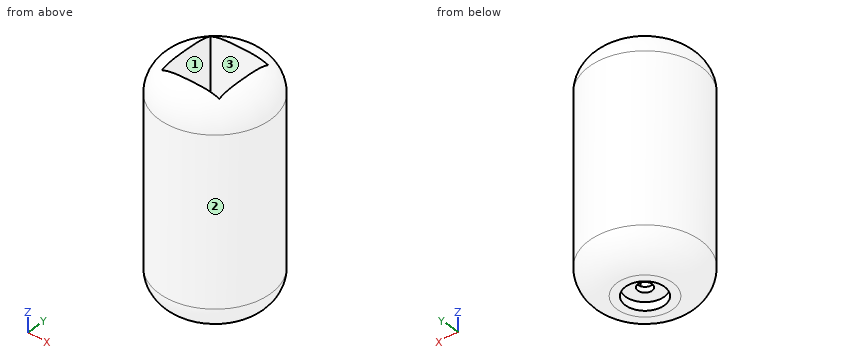
```python
from build123d import *

# Parameters (mm, degrees)
SKETCH4_R               = 20
BODY_DEPTH              = 80
CUT_EXTRUDE1_DEPTH      = 50
CUT_EXTRUDE1_DEPTH_BACK = 50
SKETCH16_W              = 21
SKETCH16_H              = 21
SKETCH17_R              = 2.55
CUT_EXTRUDE2_DEPTH      = 55
SKETCH18_R              = 7
CUT_EXTRUDE3_DEPTH      = 3
FILLET1_R               = 10


with BuildPart() as part:
    # Sketch4 → Body (new body)
    with BuildSketch(Plane.XY.offset(25)):
        Circle(SKETCH4_R)
    extrude(amount=-BODY_DEPTH)

    # Sketch16 → Cut-Extrude1 (cut, two sides: drawn at the far end of the back side and taken through both)
    with BuildSketch(Plane.XY.offset(-CUT_EXTRUDE1_DEPTH_BACK)):
        Rectangle(SKETCH16_W, SKETCH16_H)
    extrude(amount=CUT_EXTRUDE1_DEPTH + CUT_EXTRUDE1_DEPTH_BACK, mode=Mode.SUBTRACT)

    # Sketch17 → Cut-Extrude2 (cut)
    with BuildSketch(Plane(origin=(0, 0, -55), x_dir=(-1, 0, 0), z_dir=(0, 0, -1))):
        Circle(SKETCH17_R)
    extrude(amount=-CUT_EXTRUDE2_DEPTH, mode=Mode.SUBTRACT)

    # Sketch18 → Cut-Extrude3 (cut)
    with BuildSketch(Plane(origin=(0, 0, -55), x_dir=(-1, 0, 0), z_dir=(0, 0, -1))):
        Circle(SKETCH18_R)
    extrude(amount=-CUT_EXTRUDE3_DEPTH, mode=Mode.SUBTRACT)

    # Fillet1
    # the kernel refuses this fillet: 10 mm, written as the material it takes off along each edge
    with BuildSketch(Plane(origin=(0, 0, 25), x_dir=(1, 0, 0), z_dir=(0, -1, 0))) as fillet1_piece_1:
        with BuildLine():
            CenterArc((20 - FILLET1_R, -FILLET1_R), FILLET1_R, 0, 90)
            Line((20 - FILLET1_R, 0), (20, 0))
            Line((20, 0), (20, -FILLET1_R))
        make_face()
    revolve(axis=Axis((0, 0, 25), (0, 0, 1)), mode=Mode.SUBTRACT)
    with BuildSketch(Plane(origin=(0, 0, -55), x_dir=(1, 0, 0), z_dir=(0, -1, 0))) as fillet1_piece_2:
        with BuildLine():
            CenterArc((20 - FILLET1_R, FILLET1_R), FILLET1_R, 270, 90)
            Line((20 - FILLET1_R, 0), (20, 0))
            Line((20, 0), (20, FILLET1_R))
        make_face()
    revolve(axis=Axis((0, 0, -55), (0, 0, 1)), mode=Mode.SUBTRACT)


solid = part.part
```
Geometry check sheet. Reference: the model listing, model coordinates, mm. Face numbers are marked on the shaded views. Coordinates: 2 decimals unless noted, no trailing zeros. Order: outer loops, then holes, each group sorted by start corner. A loop starts at its lowest first (then second) coordinate and runs counter-clockwise, first axis right, second up.
Q1. Draft check along Y on the marked faces 1, 2 and 3. Enter one of: released by +Y, released by -Y, zero draft, split by the parting line, or undercut.
Reply:
face 1: undercut
face 2: split by the parting line
face 3: undercut
Q2. Depth check by flat-ended pin: pin 1 Ø4 at (x, z) = (0.5, 15.5) entering from -Y; pin 2 Ø12.5 at (x, y) = (0, 0) entering from -Z; pin 3 Ø3 at (y, z) = (-13, -1) entering from -X. Enter the tip coordinate at first touch or a pass-through.
Reply:
pin 1: stops at y = -20
pin 2: stops at z = -52
pin 3: stops at x = -16.36
Q3. Sectioned sample at A-A on z = -6. Record the cut outline in (x, y).
Reply:
outline: circle Ø40 at (0, 0); hole (-10.5, -10.5) - (10.5, -10.5) - (10.5, 10.5) - (-10.5, 10.5) - close
Q4. Thickness scan on probe 1 along Y at (x, z) = (0, 4.5); probe 2 along Y at (x, z) = (0, -52.9); probe 3 along X at (y, z) = (7, -35) (3 decimals). Record the ranges inside material, lowest first.
Reply:
probe 1: y = -20 to -10.5, 10.5 to 20
probe 2: y = -16.13 to -7, 7 to 16.13
probe 3: x = -18.735 to -10.5, 10.5 to 18.735
